Can you work these out from the model? Positions are in its coordinate system, mm. Face numbers are marked on the shaded views. A direction names the side the tool comes from. Coordinates: 2 decimals unless noted, no trailing zeros. Loops run counter-clockwise (first coordinate to the right, second up) from the corner with the lowest first, then second, coordinate; pieces in that order, holes last. Notation, with made-up numbers: (0, 30.25) - (5, 30.25) arc R24 cw to (5, 45.25) - close; hole circle Ø3 at (40, 38.5). An arc over 180 degrees is marked (long way). Put each result on its own line as item: value. Start each with the question number.
from build123d import *

# Parameters (mm, degrees)
SKETCH_1_R          = 21
EXTRUDE_1_DEPTH     = 32
SKETCH_2_R          = 30
EXTRUDE_2_DEPTH     = 13
SKETCH_3_R          = 14
CUT_EXTRUDE_1_DEPTH = 46
CHAMFER_1_SIZE      = 1.5


with BuildPart() as part:
    # 草图1 → 凸台-拉伸1 (new body)
    with BuildSketch(Plane(origin=(0, 0, 0), x_dir=(1, 0, 0), z_dir=(0, 1, 0))):
        Circle(SKETCH_1_R)
    extrude(amount=EXTRUDE_1_DEPTH)

    # 草图2 → 凸台-拉伸2 (add)
    with BuildSketch(Plane(origin=(0, 32, 0), x_dir=(1, 0, 0), z_dir=(0, 1, 0))):
        Circle(SKETCH_2_R)
    extrude(amount=EXTRUDE_2_DEPTH)

    # 草图3 → 切除-拉伸1 (cut, through all)
    with BuildSketch(Plane(origin=(0, 45, 0), x_dir=(1, 0, 0), z_dir=(0, 1, 0))):
        Circle(SKETCH_3_R)
    extrude(amount=-CUT_EXTRUDE_1_DEPTH, mode=Mode.SUBTRACT)

    # 倒角1
    chamfer_1_edges = [part.edges().sort_by_distance(p)[0] for p in [
        (-14, 0, 0),
        (-14, 45, 0),
        (-21, 0, 0),
        (-30, 32, 0),
        (-30, 45, 0),
    ]]
    chamfer(chamfer_1_edges, length=CHAMFER_1_SIZE)


solid = part.part
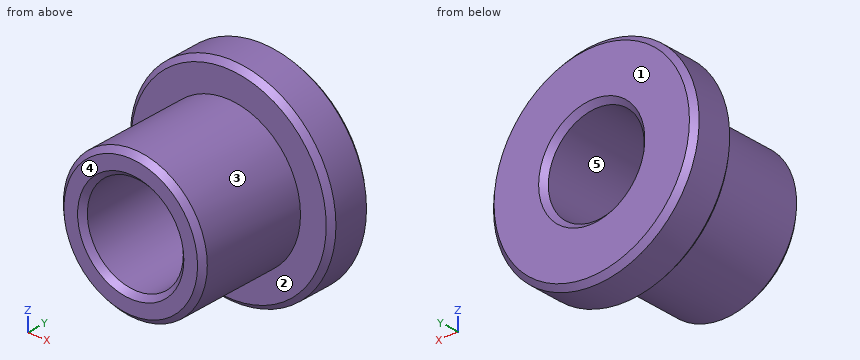
Q1. I want a section at A-A on z = 0. List the corners of the cut face in (x, y) for me.
Q2. I want a section at C-C on y = 24.5. List the corners of the cut face in (x, z) for me.
Q3. We'd pull the mould along Z, two halves only. Please class the marked faces 3, 4 and 5: released by +Z, released by -Z, zero draft, split by the parting line, or undercut.
Q4. Will these pins go through, and if not, where does the flat tip stop? pin 1 (5 mm diameter, centred on x = 13, y = 34, fed in from -Z); pin 2 (1.5 mm diameter, centred on x = 1, y = 24, fed in from +Z); pin 3 (6 mm diameter, centred on x = 5.5, y = 36.5, fed in from -Z).
Q5. I want a section at B-B on x = 0. List the corners of the cut face in (y, z) for me.
Q6. On a 3-axis mill with a long thin cutter (end or side, diameter ignored), from which of +Z, -Z, +X, -X, +Y, -Y can I reach the whole of each face in a straight line? I mean the marked faces 1 and 2. Say none if no direction works.
Q7. Please list where these lines run through material, in increasing order: line 1 along X through (y, z) = (29, 0); line 2 along X through (y, z) = (35, 0). Write a range as [from, to].
Q8. I want a section at D-D on y = 42.5. List the corners of the cut face in (x, z) for me.
Calculated:
1. outline: (-30, 33.5) - (-28.5, 32) - (-21, 32) - (-21, 1.5) - (-19.5, 0) - (-15.5, 0) - (-14, 1.5) - (-14, 43.5) - (-15.5, 45) - (-28.5, 45) - (-30, 43.5) - close; (14, 1.5) - (15.5, 0) - (19.5, 0) - (21, 1.5) - (21, 32) - (28.5, 32) - (30, 33.5) - (30, 43.5) - (28.5, 45) - (15.5, 45) - (14, 43.5) - close
2. outline: circle Ø42 at (0, 0); hole circle Ø28 at (0, 0)
3. face 3: split by the parting line
3. face 4: zero draft
3. face 5: undercut
4. pin 1: z = -28.1
4. pin 2: z = 21
4. pin 3: z = -29.9
5. outline: (0, -19.5) - (1.5, -21) - (32, -21) - (32, -28.5) - (33.5, -30) - (43.5, -30) - (45, -28.5) - (45, -15.5) - (43.5, -14) - (1.5, -14) - (0, -15.5) - close; (0, 15.5) - (1.5, 14) - (43.5, 14) - (45, 15.5) - (45, 28.5) - (43.5, 30) - (33.5, 30) - (32, 28.5) - (32, 21) - (1.5, 21) - (0, 19.5) - close
6. face 1: +Z, -Z, +X, -X, +Y
6. face 2: -Y
7. line 1: [-21, -14], [14, 21]
7. line 2: [-30, -14], [14, 30]
8. outline: circle Ø60 at (0, 0); hole circle Ø28 at (0, 0)
